```python
from build123d import *

# Parameters (mm, degrees)
BOSS_EXTRUDE1_DEPTH     = 84.5
CUT_EXTRUDE1_DEPTH      = 85.998529399
CUT_EXTRUDE1_DEPTH_BACK = 85.998529399
SKETCH2_R               = 3
SKETCH2_R_2             = 2.5


with BuildPart() as part:
    # Sketch1 → Boss-Extrude1 (new, symmetric)
    with BuildSketch(Plane.XY):
        Polygon((4.5, 3.5), (6.5, 4), (6.5, 6.5), (-6.5, 6.5), (-6.5, 4), (-4.5, 3.5), (-4.5, -3.5), (-6.5, -4), (-6.5, -6.5), (6.5, -6.5), (6.5, -4), (4.5, -3.5), align=None)
    extrude(amount=BOSS_EXTRUDE1_DEPTH, both=True)

    # Sketch2 → Cut-Extrude1 (cut, two sides: drawn at the far end of the back side and taken through both)
    with BuildSketch(Plane(origin=(0, 0, 0), x_dir=(1, 0, 0), z_dir=(0, 1, 0)).offset(-CUT_EXTRUDE1_DEPTH_BACK)):
        with Locations(Location((0, 75.5, 0), (0, 0, 270))):
            Circle(SKETCH2_R)
        with Locations(Location((0, -75.5, 0), (0, 0, 270))):
            Circle(SKETCH2_R)
        with Locations(Location((0, -65.5, 0), (0, 0, 270))):
            Circle(SKETCH2_R_2)
        with Locations(Location((0, -57.5, 0), (0, 0, 270))):
            Circle(SKETCH2_R_2)
        with Locations(Location((0, -49.5, 0), (0, 0, 270))):
            Circle(SKETCH2_R_2)
        with Locations(Location((0, -41.5, 0), (0, 0, 270))):
            Circle(SKETCH2_R_2)
        with Locations(Location((0, -33.5, 0), (0, 0, 270))):
            Circle(SKETCH2_R_2)
        with Locations(Location((0, -25.5, 0), (0, 0, 270))):
            Circle(SKETCH2_R_2)
        with Locations(Location((0, -17.5, 0), (0, 0, 270))):
            Circle(SKETCH2_R_2)
        with Locations(Location((0, -9.5, 0), (0, 0, 270))):
            Circle(SKETCH2_R_2)
        with Locations(Location((0, -1.5, 0), (0, 0, 270))):
            Circle(SKETCH2_R_2)
        with Locations(Location((0, 6.5, 0), (0, 0, 270))):
            Circle(SKETCH2_R_2)
        with Locations(Location((0, 14.5, 0), (0, 0, 270))):
            Circle(SKETCH2_R_2)
        with Locations(Location((0, 22.5, 0), (0, 0, 270))):
            Circle(SKETCH2_R_2)
        with Locations(Location((0, 30.5, 0), (0, 0, 270))):
            Circle(SKETCH2_R_2)
        with Locations(Location((0, 38.5, 0), (0, 0, 270))):
            Circle(SKETCH2_R_2)
    extrude(amount=CUT_EXTRUDE1_DEPTH + CUT_EXTRUDE1_DEPTH_BACK, mode=Mode.SUBTRACT)


solid = part.part
```
Design review of the part built by this model. Coordinates are the model's own, in mm. Coordinates: 2 decimals unless noted, no trailing zeros. Order: outer loops, then holes, each group sorted by start corner. A loop starts at its lowest first (then second) coordinate and runs counter-clockwise, first axis right, second up.
1) Take a section at A-A, the plane z = 9.5. Give the boundary of the cut face in (x, y), and give its area (3 significant figures).
2) Clearance check with flat-ended pins moving along their axes: pin 1 (4 mm diameter, centred on x = 0, z = 1.5, fed in from -Y); pin 2 (3.5 mm diameter, centred on y = -0.5, z = 6, fed in from +X); pin 3 (1.5 mm diameter, centred on x = -5, y = 0.5, fed in from +Z); pin 4 (4 mm diameter, centred on y = -1, z = -7, fed in from -X). State where each tip first meets the part, or that it passes through.
3) Wall thickness on line 1 along X through (y, z) = (1.75, 65.5); line 2 along Z through (x, y) = (2.75, 4.75); line 3 along X through (y, z) = (-0.5, -9.5): over which ranges is each line inside the solid? List them lowest first.
4) Mouldability with a two-part tool opening along X and no side actions: class faces 1 (the flat face through (-4.5, 0, 1)), 2 (the cylindrical face through (0, 0, -25)), 3 (the flat face through (4.5, 0, 1)) as +X half, -X half, draft (parallel to the pull), parting line (faces both ways), or undercut.
5) Take a section at B-B, the plane y = -1.5. State how many separate pieces and enclosed holes the cut face has, and give its area (3 significant figures).
Returned:
1. outline: (-6.5, -6.5) - (-2.5, -6.5) - (-2.5, 6.5) - (-6.5, 6.5) - (-6.5, 4) - (-4.5, 3.5) - (-4.5, -3.5) - (-6.5, -4) - close; (2.5, -6.5) - (6.5, -6.5) - (6.5, -4) - (4.5, -3.5) - (4.5, 3.5) - (6.5, 4) - (6.5, 6.5) - (2.5, 6.5) - close
1. area: 74.0 mm2
2. pin 1: passes through
2. pin 2: stops at x = 4.5
2. pin 3: stops at z = 84.5
2. pin 4: stops at x = -4.5
3. line 1: x = -4.5 to -2.5, 2.5 to 4.5
3. line 2: z = -84.5 to -76.7, -74.3 to 74.3, 76.7 to 84.5
3. line 3: x = -4.5 to 4.5
4. face 1: -X half
4. face 2: undercut
4. face 3: +X half
5. separate pieces: 1
5. enclosed holes: 16
5. area: 1,190 mm2
